Check sheet for the modelled part. Datum: model origin and axes. Units: mm. A direction names the side the tool comes from. Give positions to 0.01 mm unless a question says otherwise; leave off trailing zeros. Write each loop counter-clockwise with the first axis right and the second up, starting at its lowest first coordinate (ties: lowest second). Pieces come first, ordered by that corner, then holes. Notation, with made-up numbers: M 47,-36.75 L 76,-36.75 A8 ccw 76,-22.75 Z; hole C -20.5,-1.5 d8. An arc over 180 degrees is marked long. One line per item, written item: value. Start each with the question number.
from build123d import *

# Parameters (mm, degrees)
LID_W               = 108.75
LID_H               = 62.54
EXTRUDE_1_DEPTH     = 2
CUT_EXTRUDE_1_REACH = 95.36
SKETCH_8_W          = 72
SKETCH_8_H          = 25.5
CUT_EXTRUDE_3_REACH = 95.36
SKETCH_15_W         = 6
SKETCH_15_H         = 6
FILLET_1_R          = 1.5
SKETCH_16_W         = 108.75
SKETCH_16_H         = 62.54
SKETCH_16_W_2       = 104.75
SKETCH_16_H_2       = 58.54
EXTRUDE_2_DEPTH     = 2
SKETCH_17_W         = 14.3
SKETCH_17_H         = 17
CUT_EXTRUDE_4_DEPTH = 4
SKETCH_18_W         = 4.1
SKETCH_18_H         = 4.5
SKETCH_18_W_2       = 4.169367978
SKETCH_18_H_2       = 4.25
EXTRUDE_3_DEPTH     = 11.6


with BuildPart() as part:
    # lid → ﾎﾞｽ - 押し出し1 (new body)
    with BuildSketch(Plane(origin=(0, 0, 0), x_dir=(1, 0, 0), z_dir=(0, 1, 0))):
        with Locations((18.405, 27.17)):
            Rectangle(LID_W, LID_H)
    extrude(amount=EXTRUDE_1_DEPTH)

    # ｽｹｯﾁ8 → ｶｯﾄ - 押し出し1 (cut, up to next)
    with BuildSketch(Plane(origin=(0, 2, 0), x_dir=(1, 0, 0), z_dir=(0, 1, 0)), mode=Mode.PRIVATE) as cut_extrude_1_sk1:
        with Locations((11.13, 22.37)):
            Rectangle(SKETCH_8_W, SKETCH_8_H)
    cut_extrude_1_tool1 = extrude(cut_extrude_1_sk1.sketch, amount=-CUT_EXTRUDE_1_REACH, mode=Mode.PRIVATE) & part.part
    add(cut_extrude_1_tool1.solids().sort_by_distance((11.13, 2, -22.37))[0], mode=Mode.SUBTRACT)

    # ｽｹｯﾁ15 → ｶｯﾄ - 押し出し3 (cut, up to next)
    with BuildSketch(Plane(origin=(0, 2, 0), x_dir=(1, 0, 0), z_dir=(0, 1, 0)), mode=Mode.PRIVATE) as cut_extrude_3_sk1:
        with Locations((41.54, 40.62)):
            Rectangle(SKETCH_15_W, SKETCH_15_H)
    cut_extrude_3_tool1 = extrude(cut_extrude_3_sk1.sketch, amount=-CUT_EXTRUDE_3_REACH, mode=Mode.PRIVATE) & part.part
    # ｽｹｯﾁ15 → ｶｯﾄ - 押し出し3 (cut, up to next)
    with BuildSketch(Plane(origin=(0, 2, 0), x_dir=(1, 0, 0), z_dir=(0, 1, 0)), mode=Mode.PRIVATE) as cut_extrude_3_sk2:
        with Locations((49.34, 40.62)):
            Rectangle(SKETCH_15_W, SKETCH_15_H)
    cut_extrude_3_tool2 = extrude(cut_extrude_3_sk2.sketch, amount=-CUT_EXTRUDE_3_REACH, mode=Mode.PRIVATE) & part.part
    add(cut_extrude_3_tool1.solids().sort_by_distance((41.54, 2, -40.62))[0], mode=Mode.SUBTRACT)
    add(cut_extrude_3_tool2.solids().sort_by_distance((49.34, 2, -40.62))[0], mode=Mode.SUBTRACT)

    # ﾌｨﾚｯﾄ1
    fillet_1_edges = [part.edges().sort_by_distance(p)[0] for p in [
        (38.54, 1, -37.62),
        (38.54, 1, -43.62),
        (44.54, 1, -43.62),
        (44.54, 1, -37.62),
        (46.34, 1, -37.62),
        (46.34, 1, -43.62),
        (52.34, 1, -43.62),
        (52.34, 1, -37.62),
    ]]
    fillet(fillet_1_edges, radius=FILLET_1_R)

    # ｽｹｯﾁ16 → ﾎﾞｽ - 押し出し2 (add)
    with BuildSketch(Plane.XZ):
        with Locations((18.405, -27.17)):
            Rectangle(SKETCH_16_W, SKETCH_16_H)
        with Locations((18.405, -27.17)):
            Rectangle(SKETCH_16_W_2, SKETCH_16_H_2, mode=Mode.SUBTRACT)
    extrude(amount=EXTRUDE_2_DEPTH)

    # ｽｹｯﾁ17 → ｶｯﾄ - 押し出し4 (cut)
    with BuildSketch(Plane(origin=(0, 2, 0), x_dir=(1, 0, 0), z_dir=(0, 1, 0))):
        with Locations((65.63, 25.9)):
            Rectangle(SKETCH_17_W, SKETCH_17_H)
    extrude(amount=-CUT_EXTRUDE_4_DEPTH, mode=Mode.SUBTRACT)

    # ｽｹｯﾁ18 → ﾎﾞｽ - 押し出し3 (add)
    with BuildSketch(Plane.XZ):
        with Locations((70.73, -36.65)):
            Rectangle(SKETCH_18_W, SKETCH_18_H)
        with Locations((70.695316011, -15.275)):
            Rectangle(SKETCH_18_W_2, SKETCH_18_H_2)
    extrude(amount=EXTRUDE_3_DEPTH)


solid = part.part
1) Cross-section at C-C (x = -26). Record the boundary of the cut face in (y, z).
2) Tool access check on faces 1 (the flat face through (49, 1, -43.62)), 2 (the flat face through (69, -3, -17.4)), 3 (the flat face through (71, -11.6, -15)), 4 (the flat face through (68.611, -6, -15)). Record the directions out of +Z, -Z, +X, -X, +Y, -Y that give a thin tool (end or side, any length) a straight path to the whole face; none if there is none.
3) Material ranges on L1, parallel to Z at x = -9, y = 0.5; L2, parallel to Z at x = -9.5, y = -0.25; L3, parallel to X at y = -1.5, z = -2, recorded low to high. Write a range as from..to.
4) Cross-section at D-D (x = -1.5). Record the boundary of the cut face in (y, z), plus the area to 3 significant figures.
5) Cross-section at B-B (z = -30.5). Record the boundary of the cut face in (x, y), plus the area to 3 significant figures.
6) Cross-section at A-A (y = -9). Record the boundary of the cut face in (x, z).
7) Draft check along X on faces 5 (the flat face through (72.78, -1.7, -9.2)), 6 (the flat face through (42, 1, -37.62)), 7 (the flat face through (-35.97, 0, -28)), 8 (the flat face through (2, -2, -57)). Enter one of: released by +X, released by -X, zero draft, split by the parting line, or undercut.
8) Gauge pin test, flat ends, axial feed: pin 1 (4.5 mm diameter, centred on x = 70.5, y = -3.5, fed in from -Z); pin 2 (0.6 mm diameter, centred on y = -0.5, z = -24, fed in from +X); pin 3 (0.6 mm diameter, centred on y = 0.5, z = -21.5, fed in from +X); pin 4 (3.5 mm diameter, centred on x = 70, y = -7, fed in from +Z). Record the tip position at first contact, or that the pin passes through.
Data:
1. outline: M -2,-58.44 L 2,-58.44 L 2,4.1 L -2,4.1 L -2,2.1 L 0,2.1 L 0,-56.44 L -2,-56.44 Z
2. face 1: +Y, -Y
2. face 2: +X, +Y, -Y
2. face 3: +Z, -Z, +X, -X, -Y
2. face 4: -Y
3. L1: z = -58.44..-35.12, -9.62..4.1
3. L2: z = -58.44..-56.44, 2.1..4.1
3. L3: x = -35.97..-33.97, 70.78..72.78
4. outline: M -2,-58.44 L 2,-58.44 L 2,-35.12 L 0,-35.12 L 0,-56.44 L -2,-56.44 Z; M -2,2.1 L 0,2.1 L 0,-9.62 L 2,-9.62 L 2,4.1 L -2,4.1 Z
4. area: 82.1 mm2
5. outline: M -35.97,-2 L -33.97,-2 L -33.97,0 L -24.87,0 L -24.87,2 L -35.97,2 Z; M 47.13,0 L 58.48,0 L 58.48,2 L 47.13,2 Z
5. area: 48.9 mm2
6. outline: M 68.61,-17.4 L 72.78,-17.4 L 72.78,-13.15 L 68.61,-13.15 Z; M 68.68,-38.9 L 72.78,-38.9 L 72.78,-34.4 L 68.68,-34.4 Z
7. face 5: released by +X
7. face 6: undercut
7. face 7: released by -X
7. face 8: zero draft
8. pin 1: stops at z = -58.44
8. pin 2: stops at x = -33.97
8. pin 3: stops at x = 58.48
8. pin 4: stops at z = -13.15
